Job drawing, mm, ordinate dimensions from the low corner. One solid piece. A direction names the side the tool comes from. Round coordinates to 2 decimals unless told otherwise and drop trailing zeros. Loops run counter-clockwise (first coordinate to the right, second up) from the corner with the lowest first, then second, coordinate; pieces in that order, holes last.
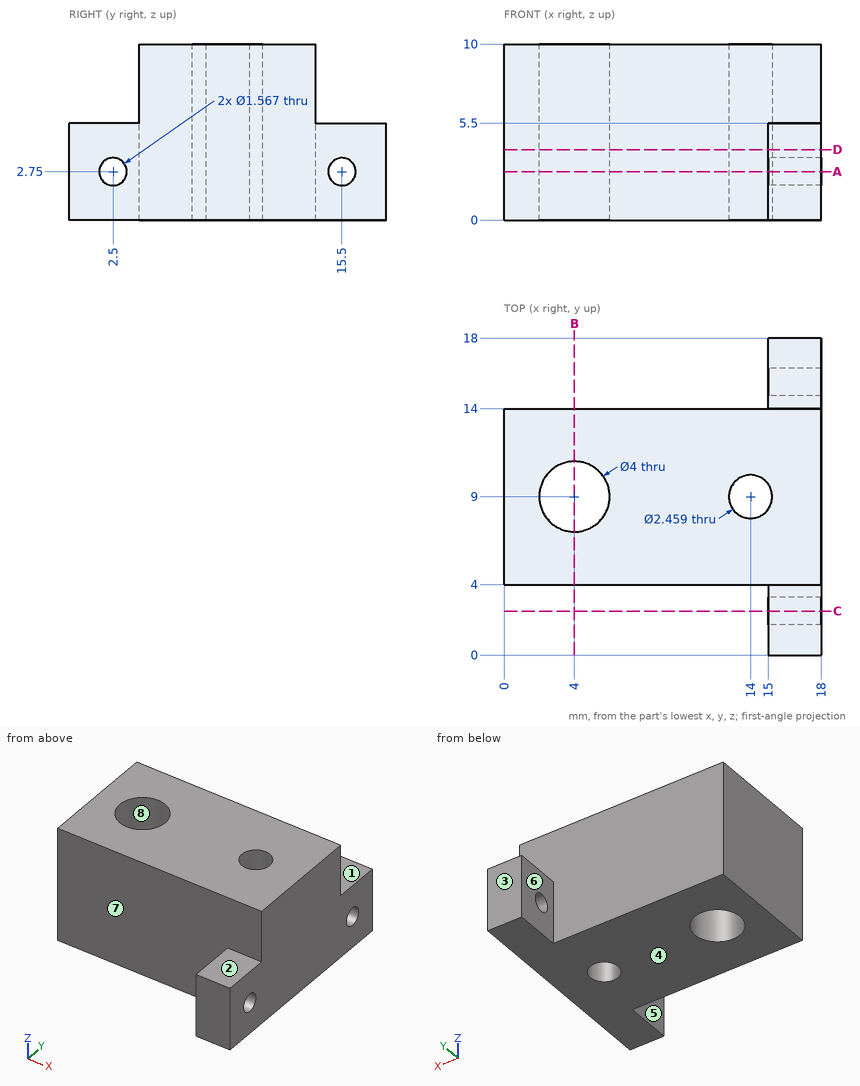
1) Slice it at C-C, the plane y = 2.5. Give the cut face in (x, z), then the cut area to 3 significant figures.
Values:
outline: (15, 0) - (18, 0) - (18, 1.97) - (15, 1.97) - close; (15, 3.53) - (18, 3.53) - (18, 5.5) - (15, 5.5) - close
area: 11.8 mm2
2) Slice it at B-B, the plane x = 4. Give the cut face in (y, z), then the cut area to 3 significant figures.
Values:
outline: (4, 0) - (7, 0) - (7, 10) - (4, 10) - close; (11, 0) - (14, 0) - (14, 10) - (11, 10) - close
area: 60.0 mm2
3) Mould opens along X. For the marked faces 6, 7 and 8 say: released by +X, released by -X, zero draft, split by the parting line, or undercut.
Values:
face 6: released by -X
face 7: zero draft
face 8: undercut
4) Drop flat-ended pins along their axis: pin 1 Ø1.5 at (x, y) = (17, 16) entering from +Z; pin 2 Ø4 at (x, z) = (7, 6) entering from +Y; pin 3 Ø6 at (x, z) = (15, 6.5) entering from +Y. Give the stop position or say it passes through.
Values:
pin 1: stops at z = 5.5
pin 2: stops at y = 14
pin 3: stops at y = 18
5) Tool access for the marked faces 1, 2, 3, 4 and 5: list every direction of +Z, -Z, +X, -X, +Y, -Y with a clear straight run to the whole face (end or side of a thin tool).
Values:
face 1: +Z, +X, -X, +Y
face 2: +Z, +X, -X, -Y
face 3: +Z, -Z, +X, -X, +Y
face 4: -Z, +X, -X, +Y, -Y
face 5: +Z, -Z, -X, -Y
6) Slice it at A-A, the plane z = 2.75. Give the cut face in (x, y).
Values:
outline: (0, 4) - (15, 4) - (15, 3.28) - (18, 3.28) - (18, 14.72) - (15, 14.72) - (15, 14) - (0, 14) - close; (15, 0) - (18, 0) - (18, 1.72) - (15, 1.72) - close; (15, 16.28) - (18, 16.28) - (18, 18) - (15, 18) - close; hole circle Ø4 at (4, 9); hole circle Ø2.46 at (14, 9)
7) Slice it at D-D, the plane z = 4. Give the cut face in (x, y), then the cut area to 3 significant figures.
Values:
outline: (0, 4) - (15, 4) - (15, 0) - (18, 0) - (18, 18) - (15, 18) - (15, 14) - (0, 14) - close; hole circle Ø4 at (4, 9); hole circle Ø2.46 at (14, 9)
area: 187 mm2
8) Wall check: line 1 along Z through (x, y) = (16, 15.5); line 2 along X through (y, z) = (9.5, 5.75); line 3 along Y through (x, z) = (14, 3.5). Give the ranges that are in metal, low to high.
Values:
line 1: z = 0 to 1.97, 3.53 to 5.5
line 2: x = 0 to 2.06, 5.94 to 12.88, 15.12 to 18
line 3: y = 4 to 7.77, 10.23 to 14
